from build123d import *

# Parameters (mm, degrees)
SKETCH1_W             = 3
SKETCH1_H             = 16
BOSS_EXTRUDE1_DEPTH   = 42.25
BOSS_EXTRUDE1_2_DEPTH = 42.25
SKETCH2_W             = 55.024264068
SKETCH2_H             = 42.424264068
BOSS_EXTRUDE2_DEPTH   = 2
SKETCH4_W             = 44.25
SKETCH4_H             = 16
SKETCH4_R             = 3.5
BOSS_EXTRUDE4_DEPTH   = 10


with BuildPart() as part:
    # Sketch1 → Boss-Extrude1 (new body)
    with BuildSketch(Plane.XY):
        with Locations((26.012132034, 0)):
            Rectangle(SKETCH1_W, SKETCH1_H)
    extrude(amount=BOSS_EXTRUDE1_DEPTH)



with BuildPart() as body_2:
    # Sketch1 → Boss-Extrude1 2 (new body)
    with BuildSketch(Plane.XY):
        with Locations((-26.012132034, 0)):
            Rectangle(SKETCH1_W, SKETCH1_H)
    extrude(amount=BOSS_EXTRUDE1_2_DEPTH)


with BuildPart() as part_1:
    add(part.part)

    add(body_2.part)  # Boss-Extrude2 merges body 2
    # Sketch2 → Boss-Extrude2 (add)
    with BuildSketch(Plane.XY.offset(42.25)):
        Rectangle(SKETCH2_W, SKETCH2_H)
    extrude(amount=BOSS_EXTRUDE2_DEPTH)

    # Sketch4 → Boss-Extrude4 (add)
    with BuildSketch(Plane(origin=(27.512132034, 0, 0), x_dir=(0, 0, -1), z_dir=(1, 0, 0))):
        with Locations((-22.125, 0)):
            Rectangle(SKETCH4_W, SKETCH4_H)
        with Locations((-22.125, 0)):
            Circle(SKETCH4_R, mode=Mode.SUBTRACT)
    extrude(amount=BOSS_EXTRUDE4_DEPTH)


solid = part_1.part
The listing builds one solid part. Answer for the finished solid, in the listing's coordinates (mm). A direction names the side the tool comes from. Give positions to 0.01 mm unless a question says otherwise; leave off trailing zeros. Write each loop counter-clockwise with the first axis right and the second up, starting at its lowest first coordinate (ties: lowest second). Pieces come first, ordered by that corner, then holes.
Item 1: Flat-ended cylindrical pins translate along their axes: P1, Ø2, axis at y = -15, z = 43, coming from the +X side; P2, Ø6, axis at x = 25, y = 13, coming from the -Z side; P3, Ø1.5, axis at x = -26.5, z = 22, coming from the +Y side. Find the tip coordinate at first contact, or state that the pin passes through.
Item 2: Section C-C, the plane x = 26.5 is taken. Write down the section's boundary in (y, z), plus the area to 3 significant figures.
Item 3: Section A-A, the plane z = 14.5 is taken. Write down the section's boundary in (x, y), plus the area to 3 significant figures.
Item 4: Find the intervals of material crossed by line 1 along X through (y, z) = (-0.5, 27); line 2 along Z through (x, y) = (-10, -5.5); line 3 along Y through (x, z) = (29.5, 30), in increasing order.
Item 5: Determine the mould class of faces 6 (the cylindrical face through (32.442, 1.051, 18.787)), 7 (the flat face through (31, -8, 22)), 8 (the flat face through (5, 0, 44.25)) for opening direction Z: released by +Z, released by -Z, zero draft, split by the parting line, or undercut.
Item 6: Section D-D, the plane z = 20.5 is taken. Write down the section's boundary in (x, y).
Item 7: Which of the six approach directions +Z, -Z, +X, -X, +Y, -Y give full straight-line access (tool end or side, diameter ignored) to faces 1 (the flat face through (27.512, -15, 43)), 2 (the flat face through (-24.512, 0, 21)), 3 (the flat face through (27.512, 0, 22)), 4 (the flat face through (27.512, 15, 43)), 5 (the flat face through (-26, 8, 21))?
Item 8: Section B-B, the plane y = 4.5 is taken. Write down the section's boundary in (x, z), plus the area to 3 significant figures.
Completed:
1. P1: stops at x = 27.51
1. P2: stops at z = 42.25
1. P3: stops at y = 8
2. outline: (-21.21, 42.25) - (-8, 42.25) - (-8, 0) - (8, 0) - (8, 42.25) - (21.21, 42.25) - (21.21, 44.25) - (-21.21, 44.25) - close
2. area: 761 mm2
3. outline: (-27.51, -8) - (-24.51, -8) - (-24.51, 8) - (-27.51, 8) - close; (24.51, -8) - (37.51, -8) - (37.51, 8) - (24.51, 8) - close
3. area: 256 mm2
4. line 1: x = -27.51 to -24.51, 24.51 to 37.51
4. line 2: z = 42.25 to 44.25
4. line 3: y = -8 to 8
5. face 6: undercut
5. face 7: zero draft
5. face 8: released by +Z
6. outline: (-27.51, -8) - (-24.51, -8) - (-24.51, 8) - (-27.51, 8) - close; (24.51, -8) - (37.51, -8) - (37.51, -3.1) - (27.51, -3.1) - (27.51, 3.1) - (37.51, 3.1) - (37.51, 8) - (24.51, 8) - close
7. face 1: +Z, -Z, +X, -Y
7. face 2: -Z, +Y, -Y
7. face 3: +X
7. face 4: +Z, -Z, +X, +Y
7. face 5: -Z, +X, -X, +Y
8. outline: (-27.51, 0) - (-24.51, 0) - (-24.51, 42.25) - (24.51, 42.25) - (24.51, 0) - (37.51, 0) - (37.51, 44.25) - (-27.51, 44.25) - close
8. area: 806 mm2
